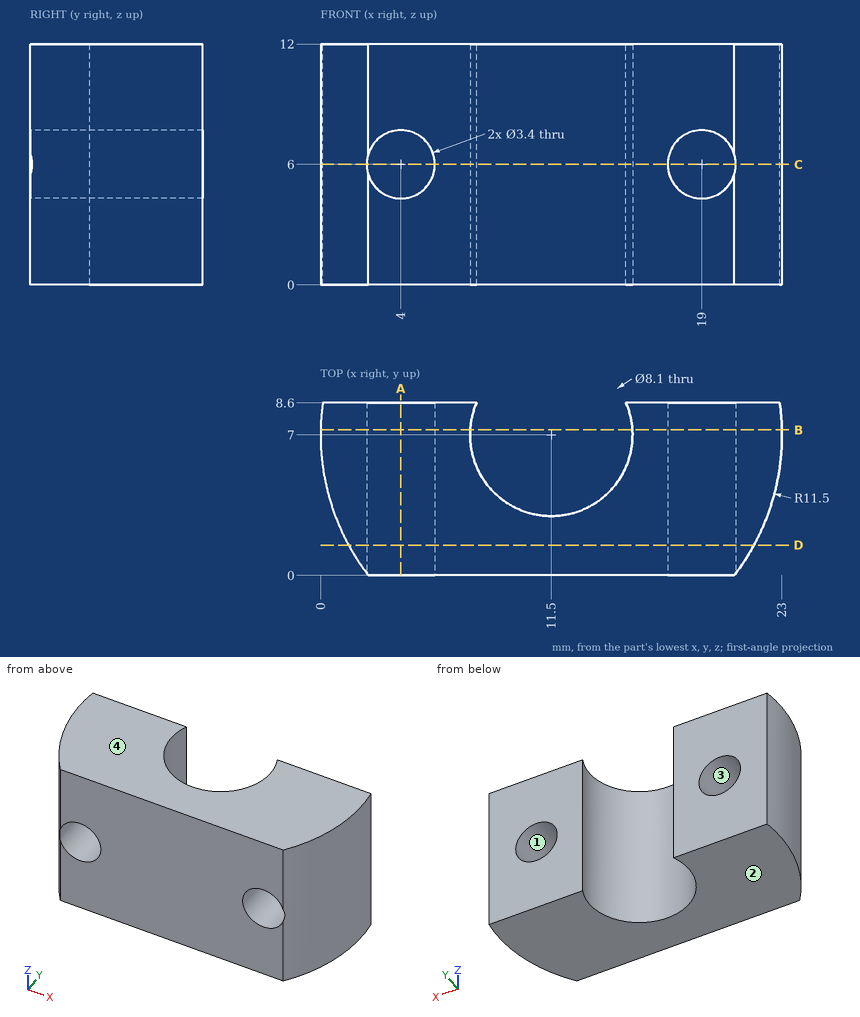
Study the drawing (mm; zero at the part's minimum x, y, z) and answer. Give positions to 0.01 mm unless a question says otherwise; leave off trailing zeros. Loops run counter-clockwise (first coordinate to the right, second up) from the corner with the lowest first, then second, coordinate; pieces in that order, holes last. Notation, with made-up numbers: (59, 17.5) -> (85, 17.5) arc R19 cw to (85, 49.5) -> close; hole circle Ø3 at (38.5, -10). An arc over 180 degrees is marked (long way). Use a Markdown table: item, result. Add a question column.
1) The part is cut by section D-D, the plane y = 1.5. Determine the outline of the cut face in (x, z).
2) Consider line 1 along X through (y, z) = (1.25, 4.5); line 2 along X through (y, z) = (4.25, 6); line 3 along X through (y, z) = (6.25, 5). Determine where each line is inside the solid, lowest interval first.
3) The part is cut by section C-C, the plane z = 6. Determine the outline of the cut face in (x, y).
4) Each of these flat-tipped pins is pushed along its axis until it touches: P1, Ø4, axis at y = 6.5, z = 6.5, coming from the +X side; P2, Ø2, axis at x = 4, z = 6, coming from the -Y side. Where does it stop, or does it pass through?
5) The part is cut by section A-A, the plane x = 4. Determine the outline of the cut face in (y, z).
6) For a pull along Z with two mould halves and no side action, classify the marked faces 1, 2, 3 and 4 as +Z half, -Z half, draft (parallel to the pull), parting line (faces both ways), or undercut.
7) The part is cut by section B-B, the plane y = 7.25. Determine the outline of the cut face in (x, z), plus the area to 3 significant figures.
Reported:
| question | item | result |
|---|---|---|
| 1 | outline | (1.4, 0) -> (21.6, 0) -> (21.6, 12) -> (1.4, 12) -> close; hole circle Ø3.4 at (4, 6); hole circle Ø3.4 at (19, 6) |
| 2 | line 1 | x = 1.54 to 3.2, 4.8 to 18.2, 19.8 to 21.46 |
| 2 | line 2 | x = 0.33 to 2.3, 5.7 to 8.53, 14.47 to 17.3, 20.7 to 22.67 |
| 2 | line 3 | x = 0.02 to 2.63, 5.37 to 7.52, 15.48 to 17.63, 20.37 to 22.98 |
| 3 | outline | (0.11, 8.6) arc R11.5 ccw to (2.3, 0.1) -> (2.3, 8.6) -> close; (5.7, 0) -> (17.3, 0) -> (17.3, 8.6) -> (15.22, 8.6) arc R4.05 cw (long way) to (7.78, 8.6) -> (5.7, 8.6) -> close; (20.7, 0.1) arc R11.5 ccw to (22.89, 8.6) -> (20.7, 8.6) -> close |
| 4 | P1 | stops at x = 23 |
| 4 | P2 | passes through |
| 5 | outline | (0, 0) -> (8.6, 0) -> (8.6, 4.3) -> (0, 4.3) -> close; (0, 7.7) -> (8.6, 7.7) -> (8.6, 12) -> (0, 12) -> close |
| 6 | face 1 | undercut |
| 6 | face 2 | -Z half |
| 6 | face 3 | undercut |
| 6 | face 4 | +Z half |
| 7 | outline | (0, 0) -> (7.46, 0) -> (7.46, 12) -> (0, 12) -> close; (15.54, 0) -> (23, 0) -> (23, 12) -> (15.54, 12) -> close; hole circle Ø3.4 at (4, 6); hole circle Ø3.4 at (19, 6) |
| 7 | area | 161 mm^2 |
